Check sheet for the modelled part. Datum: model origin and axes. Units: mm. Face numbers are marked on the shaded views. A direction names the side the tool comes from. Give positions to 0.01 mm unless a question says otherwise; leave off trailing zeros. Write each loop counter-clockwise with the first axis right and the second up, starting at its lowest first coordinate (ties: lowest second). Pieces come first, ordered by that corner, then holes. Notation, with made-up numbers: M 32,29.5 L 60,29.5 A30 cw 60,53.5 Z; hole C 88,-35.75 d5. An arc over 180 degrees is marked long. Write item = value, one per line. Start each with the question number.
1) Scan lines: line 1 along X through (y, z) = (3, -18); line 2 along X through (y, z) = (5.9, -20.45); line 3 along X through (y, z) = (6.5, -23.25). Record each from-to range of solid material in increasing order. Write a range as [from, to].
2) Mould release check, pull along Z, two halves, no side actions. Record for the marked faces 1, 2, 3 and 4: released by +Z, released by -Z, zero draft, split by the parting line, or undercut.
3) Cross-section at D-D, the plane x = 3.5. Record the cut outline in (y, z).
4) Access from +Z, -Z, +X, -X, +Y, -Y to the whole of each face (thin tool, end or side, straight path). Record for the marked faces 5 and 6.
5) Go/stop test with flat-tipped pins: pin 1 (2 mm diameter, centred on x = -0.5, y = 4, fed in from +Z); pin 2 (1 mm diameter, centred on x = 0, y = -1, fed in from +Z); pin 3 (2 mm diameter, centred on x = -13.5, z = -6, fed in from +Y). Record where each tip stops, or that it passes through.
6) Cross-section at C-C, the plane z = 19.45. Record the cut outline in (x, y).
7) Cross-section at A-A, the plane y = 6.75. Record the cut outline in (x, z), plus the area to 3 significant figures.
8) Cross-section at B-B, the plane y = 2.5. Record the cut outline in (x, z).
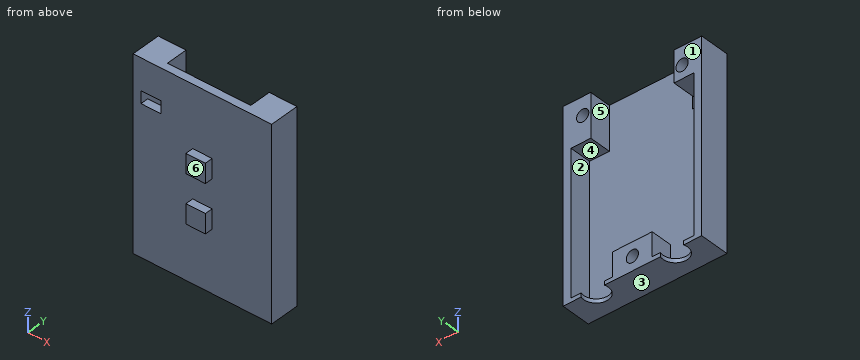
```python
from build123d import *

# Parameters (mm, degrees)
SKETCH1_W           = 35
SKETCH1_H           = 48
BOSS_EXTRUDE1_DEPTH = 2
SKETCH2_W           = 35
SKETCH2_H           = 48
SKETCH2_W_2         = 31
SKETCH2_H_2         = 44
BOSS_EXTRUDE2_DEPTH = 5.5
SKETCH3_W           = 10
SKETCH3_H           = 6
SKETCH3_W_2         = 5
SKETCH3_H_2         = 8
BOSS_EXTRUDE3_DEPTH = 5.5
SKETCH4_W           = 21
SKETCH4_H           = 5.5
CUT_EXTRUDE1_DEPTH  = 3
SKETCH5_W           = 4.9
SKETCH5_H           = 4.9
BOSS_EXTRUDE4_DEPTH = 2
CUT_EXTRUDE2_DEPTH  = 2
CUT_EXTRUDE3_START  = -7.5
SKETCH7_W           = 5
SKETCH7_H           = 3.1
CUT_EXTRUDE3_DEPTH  = 7.5
CUT_EXTRUDE4_START  = 7.5
SKETCH8_R           = 1.55
CUT_EXTRUDE4_DEPTH  = 5.5


with BuildPart() as part:
    # Sketch1 → Boss-Extrude1 (new body)
    with BuildSketch(Plane(origin=(0, 0, 0), x_dir=(1, 0, 0), z_dir=(0, 1, 0))):
        Rectangle(SKETCH1_W, SKETCH1_H)
    extrude(amount=BOSS_EXTRUDE1_DEPTH)

    # Sketch2 → Boss-Extrude2 (add)
    with BuildSketch(Plane(origin=(0, 2, 0), x_dir=(1, 0, 0), z_dir=(0, 1, 0))):
        Rectangle(SKETCH2_W, SKETCH2_H)
        with Locations((0, 1)):
            Rectangle(SKETCH2_W_2, SKETCH2_H_2, mode=Mode.SUBTRACT)
    extrude(amount=BOSS_EXTRUDE2_DEPTH)

    # Sketch3 → Boss-Extrude3 (add)
    with BuildSketch(Plane(origin=(0, 2, 0), x_dir=(1, 0, 0), z_dir=(0, 1, 0))):
        with Locations((0, 20)):
            Rectangle(SKETCH3_W, SKETCH3_H)
        with Locations((-13, -17)):
            Rectangle(SKETCH3_W_2, SKETCH3_H_2)
        with Locations((13, -17)):
            Rectangle(SKETCH3_W_2, SKETCH3_H_2)
    extrude(amount=BOSS_EXTRUDE3_DEPTH)

    # Sketch4 → Cut-Extrude1 (cut)
    with BuildSketch(Plane.XY.offset(24)):
        with Locations((0, 4.75)):
            Rectangle(SKETCH4_W, SKETCH4_H)
    extrude(amount=-CUT_EXTRUDE1_DEPTH, mode=Mode.SUBTRACT)

    # Sketch5 → Boss-Extrude4 (add)
    with BuildSketch(Plane.XZ):
        with Locations((0, 6.05)):
            Rectangle(SKETCH5_W, SKETCH5_H)
        with Locations((0, -6.05)):
            Rectangle(SKETCH5_W, SKETCH5_H)
    extrude(amount=BOSS_EXTRUDE4_DEPTH)

    # Sketch6 → Cut-Extrude2 (cut)
    with BuildSketch(Plane(origin=(0, 0, -24), x_dir=(-1, 0, 0), z_dir=(0, 0, -1))):
        with BuildLine():
            ThreePointArc((-12.93428015, 7.5), (-10, 3.4), (-7.06571985, 7.5))
            Line((-7.06571985, 7.5), (-12.93428015, 7.5))
        make_face()
        with BuildLine():
            Line((12.93428015, 7.5), (7.06571985, 7.5))
            ThreePointArc((7.06571985, 7.5), (10, 3.4), (12.93428015, 7.5))
        make_face()
    extrude(amount=-CUT_EXTRUDE2_DEPTH, mode=Mode.SUBTRACT)

    # Sketch7 → Cut-Extrude3 (cut)
    with BuildSketch(Plane(origin=(0, 7.5, 0), x_dir=(1, 0, 0), z_dir=(0, 1, 0)).offset(CUT_EXTRUDE3_START)):
        with Locations((-13, -14.55)):
            Rectangle(SKETCH7_W, SKETCH7_H)
    extrude(amount=CUT_EXTRUDE3_DEPTH, mode=Mode.SUBTRACT)

    # Sketch8 → Cut-Extrude4 (cut)
    with BuildSketch(Plane(origin=(0, 0, 0), x_dir=(1, 0, 0), z_dir=(0, 1, 0)).offset(CUT_EXTRUDE4_START)):
        with Locations(Location((-12.55, -19.45, 0), (0, 0, 270))):
            Circle(SKETCH8_R)
        with Locations(Location((12.55, -19.45, 0), (0, 0, 270))):
            Circle(SKETCH8_R)
        with Locations(Location((0, 20.45, 0), (0, 0, 270))):
            Circle(SKETCH8_R)
    extrude(amount=-CUT_EXTRUDE4_DEPTH, mode=Mode.SUBTRACT)


solid = part.part
```
Reply:
q1.line_1 = [-17.5, -15.5], [-5, 5], [15.5, 17.5]
q1.line_2 = [-17.5, -15.5], [-5, -1.55], [1.55, 5], [15.5, 17.5]
q1.line_3 = [-17.5, -13.1], [-6.9, 6.9], [13.1, 17.5]
q2.face_1 = zero draft
q2.face_2 = undercut
q2.face_3 = released by -Z
q2.face_4 = undercut
q3.outline = M 0,-24 L 7.5,-24 L 7.5,-17 L 2,-17 L 2,24 L 0,24 Z
q4.face_5 = +Z, +Y
q4.face_6 = +Z, -Z, +X, -X, -Y
q5.pin_1 = -17
q5.pin_2 = 8.5
q5.pin_3 = 2
q6.outline = M -17.5,0 L 17.5,0 L 17.5,7.5 L 14.1,7.5 L 14.1,2 L 11,2 L 11,7.5 L 10.5,7.5 L 10.5,2 L -10.5,2 L -10.5,7.5 L -11,7.5 L -11,2 L -14.1,2 L -14.1,7.5 L -17.5,7.5 Z
q7.outline = M -17.5,-24 L -13.09,-24 L -13.09,-23 L -15.5,-23 L -15.5,16.1 L -10.5,16.1 L -10.5,24 L -17.5,24 Z; M -6.91,-24 L 6.91,-24 L 6.91,-23 L 5,-23 L 5,-17 L -5,-17 L -5,-23 L -6.91,-23 Z; M 10.5,13 L 15.5,13 L 15.5,-23 L 13.09,-23 L 13.09,-24 L 17.5,-24 L 17.5,24 L 10.5,24 Z; hole C -12.55,19.45 d3.1; hole C 0,-20.45 d3.1; hole C 12.55,19.45 d3.1
q7.area = 342 mm2
q8.outline = M -17.5,-24 L 17.5,-24 L 17.5,24 L 10.5,24 L 10.5,13 L 15.5,13 L 15.5,-23 L 5,-23 L 5,-17 L -5,-17 L -5,-23 L -15.5,-23 L -15.5,16.1 L -10.5,16.1 L -10.5,24 L -17.5,24 Z; hole C -12.55,19.45 d3.1; hole C 0,-20.45 d3.1; hole C 12.55,19.45 d3.1
